```python
from build123d import *

# Parameters (mm, degrees)
F0_W      = 90
F0_H      = 170
F1_DEPTH  = 4
F2_W      = 50
F2_H      = 170
F3_DEPTH  = 4
F4_W      = 50
F4_H      = 170
F5_DEPTH  = 4
F6_DEPTH  = 4
F9_D      = 27
F13_DEPTH = 88.2
F15_DEPTH = 87.7
F16_DEPTH = 1.4
F21_DEPTH = 50
F23_DEPTH = 50
F25_DEPTH = 50


with BuildPart() as f1:
    # F0 (on Front) → F1 (new body)
    with BuildSketch(Plane.XZ):
        with Locations((10.9441001713, -7.0722334087)):
            Rectangle(F0_W, F0_H)
    extrude(amount=F1_DEPTH)

    # F2 (on face) → F3 (join)
    with BuildSketch(Plane.YZ.offset(55.9441001713)):
        with Locations((-29, -7.0722334087)):
            Rectangle(F2_W, F2_H)
    extrude(amount=-F3_DEPTH)


with BuildPart() as f5:
    # F4 (on face) → F5 (new body)
    with BuildSketch(Plane(origin=(-34.0558998287, 0, 0), x_dir=(0, -1, 0), z_dir=(-1, 0, 0))):
        with Locations((29, -7.0722334087)):
            Rectangle(F4_W, F4_H)
    extrude(amount=F5_DEPTH)


with BuildPart() as f6:
    # F6 (new): a face of the model
    f6_faces = [f5.part.faces().sort_by_distance(p)[0] for p in [
        (-36.0558998287, -4, -7.0722334087),
    ]]
    extrude(f6_faces, amount=F6_DEPTH)


with BuildPart() as f1_1:
    add(f1.part)

    # F7: union F6, F5
    add(f6.part)
    add(f5.part)

    # F9 (through all)
    with Locations(Plane.YZ.offset(55.9441001713)):
        with Locations((-27, 21.9277665913)):
            Hole(F9_D / 2)

    # F12 (on face) → F13 (join)
    with BuildSketch(Plane.YZ.offset(-34.0558998287)):
        Polygon((-38.1409525871, 60.4024082422), (-53.344592452, 66.2663727999), (-53.344592452, 63.0900636315), (-38.1409525871, 57.2260990739), align=None)
    extrude(amount=F13_DEPTH)

    # F14 (on face) → F15 (join)
    with BuildSketch(Plane.YZ.offset(-34.0558998287)):
        Polygon((-5.4573006312, 61.4672620258), (-4.8942677677, 66.4745345712), (-16.1511674523, 57.9817742109), (-13.9479605441, 55.0614893921), align=None)
    extrude(amount=F15_DEPTH)

    # F16 (add): a face of the model
    f16_faces = [f1_1.faces().sort_by_distance(p)[0] for p in [
        (8.9441001713, -15.0495639982, 56.5216318015),
    ]]
    extrude(f16_faces, amount=F16_DEPTH)

    # F20 (on face) → F21 (join)
    with BuildSketch(Plane.XZ.offset(4)):
        Polygon((10.2237635952, -25.2774868811), (-33.625573637, 7.9224472197), (-33.625573637, 3.9224472197), (10.2237635952, -29.2774868811), align=None)
    extrude(amount=F21_DEPTH)

    # F22 (on face) → F23 (join)
    with BuildSketch(Plane.XZ.offset(4)):
        Polygon((55.5519397916, -16.0052882843), (55.5519397916, -12.0052882843), (11.254648678, -42.0052882843), (11.254648678, -46.0052882843), align=None)
    extrude(amount=F23_DEPTH)

    # F24 (on face) → F25 (join)
    with BuildSketch(Plane.XZ.offset(4)):
        Polygon((5.6939503777, -62.7291997522), (-33.4860496223, -32.7291997522), (-33.4860496223, -36.7291997522), (5.6939503777, -66.7291997522), (10.9179503777, -70.7291997522), (10.9179503777, -66.7291997522), align=None)
    extrude(amount=F25_DEPTH)


solid = f1_1.part
```
Can you work these out from the model? Positions are in its coordinate system, mm. A direction names the side the tool comes from. Coordinates: 2 decimals unless noted, no trailing zeros. Loops run counter-clockwise (first coordinate to the right, second up) from the corner with the lowest first, then second, coordinate; pieces in that order, holes last.
Item 1: Suppose I cut it at B-B (x = 16.5). Please give me the cut outline in (y, z), then the cut area to 3 significant figures.
Answers below:
outline: (-54, -42.45) - (-4, -42.45) - (-4, -92.07) - (0, -92.07) - (0, 77.93) - (-4, 77.93) - (-4, -38.45) - (-54, -38.45) - close; (-53.34, 63.09) - (-38.14, 57.23) - (-38.14, 60.4) - (-53.34, 66.27) - close; (-17.27, 57.14) - (-15.07, 54.22) - (-5.46, 61.47) - (-4.89, 66.47) - close
area: 979 mm2
Item 2: If we mould it in two halves opening along X, with no side actions, what happens to faces 4 (the face through (10, 0, -8)), 5 (the face through (8, -38.141, 59)), 6 (the face through (11.255, -29, -44)), 7 (the face through (55.944, -27, -6))? For each: released by +X, released by -X, zero draft, split by the parting line, or undercut.
Answers below:
face 4: zero draft
face 5: undercut
face 6: undercut
face 7: released by +X
Item 3: I'm going to push flat-ended pins straight in: pin 1 (2.5 mm diameter, centred on x = 8.5, z = 64, fed in from -Y); pin 2 (2 mm diameter, centred on x = -27.5, y = -10, fed in from +Z); pin 3 (1 mm diameter, centred on x = -6, z = 59, fed in from +Y); pin 4 (2 mm diameter, centred on x = 8, y = -48.5, fed in from -Z). Where does each tip first touch, or does it pass through?
Answers below:
pin 1: stops at y = -53.34
pin 2: stops at z = 63.38
pin 3: stops at y = 0
pin 4: stops at z = -69.26
Item 4: Which directions (+Z, -Z, +X, -X, +Y, -Y) give clear straight access to the entire face, cutting with the end or side of a thin tool? Please do faces 1 (the face through (8.342, -45.636, 63.293)), 2 (the face through (-10.97, -28.65, -49.97)), 3 (the face through (-11.595, -28.65, -53.491)).
Answers below:
face 1: +Z
face 2: -Y
face 3: -Z, -Y
Item 5: Suppose I cut it at C-C (y = -48). Please give me the cut outline in (x, z) (3 decimals).
Answers below:
outline: (-38.056, -92.072) - (-34.056, -92.072) - (-34.056, 61.029) - (51.944, 61.029) - (51.944, -14.449) - (11.255, -42.005) - (11.255, -46.005) - (51.944, -18.449) - (51.944, -92.072) - (55.944, -92.072) - (55.944, 77.928) - (51.944, 77.928) - (51.944, 64.205) - (-34.056, 64.205) - (-34.056, 77.928) - (-38.056, 77.928) - close; (-33.626, 3.922) - (10.224, -29.277) - (10.224, -25.277) - (-33.626, 7.922) - close; (-33.486, -36.729) - (10.918, -70.729) - (10.918, -66.729) - (-33.486, -32.729) - close
Item 6: Please list where these lines run through material, in increasing order: L1, parallel to Z at x = -36, y = -27; L2, parallel to X at y = -6.5, z = -58.5; L3, parallel to X at y = -35, z = -77.
Answers below:
L1: z = -92.07 to 8.43, 35.43 to 77.93
L2: x = -38.06 to -34.06, -5.05 to 0.17, 51.94 to 55.94
L3: x = -38.06 to -34.06, 51.94 to 55.94
Item 7: Suppose I cut it at D-D (z = -35). Please give me the cut outline in (x, y), then the cut area to 3 significant figures.
Answers below:
outline: (-38.06, -54) - (-34.06, -54) - (-34.06, -4) - (-33.49, -4) - (-33.49, -54) - (-30.52, -54) - (-30.52, -4) - (21.6, -4) - (21.6, -54) - (27.5, -54) - (27.5, -4) - (51.94, -4) - (51.94, -54) - (55.94, -54) - (55.94, 0) - (-38.06, 0) - close
area: 1,220 mm2
Item 8: Suppose I cut it at A-A (y = -27). Please give me the cut outline in (x, z).
Answers below:
outline: (-38.06, -92.07) - (-34.06, -92.07) - (-34.06, 8.43) - (-38.06, 8.43) - close; (-38.06, 35.43) - (-34.06, 35.43) - (-34.06, 77.93) - (-38.06, 77.93) - close; (-33.63, 3.92) - (10.22, -29.28) - (10.22, -25.28) - (-33.63, 7.92) - close; (-33.49, -36.73) - (10.92, -70.73) - (10.92, -66.73) - (-33.49, -32.73) - close; (11.25, -46.01) - (51.94, -18.45) - (51.94, -92.07) - (55.94, -92.07) - (55.94, 8.43) - (51.94, 8.43) - (51.94, -14.45) - (11.25, -42.01) - close; (51.94, 35.43) - (55.94, 35.43) - (55.94, 77.93) - (51.94, 77.93) - close
